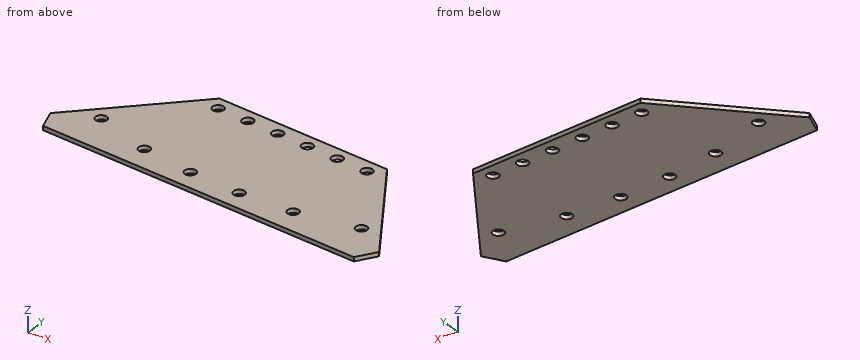
Autodesk Inventor part; units mm, degrees
ref_plane "YZ Plane" through (0, 0, 0) normal (1, 0, 0) x (0, 1, 0)
ref_plane "XZ Plane" through (0, 0, 0) normal (0, 1, 0) x (-1, 0, 0)
ref_plane "XY Plane" through (0, 0, 0) normal (0, 0, 1) x (1, 0, 0)
sketch "Sketch1" plane through (0, 0, 0) normal (0, 0, 1) x (1, 0, 0)
  circle A0 centre (31.6038, 86.1786) radius 2.1844
  circle A1 centre (18.9769, 87.5393) radius 2.1844
  circle A2 centre (6.35, 88.9) radius 2.1844
  circle A3 centre (-6.2769, 90.2607) radius 2.1844
  circle A4 centre (-18.9038, 91.6214) radius 2.1844
  circle A5 centre (-31.5307, 92.9821) radius 2.1844
  line L0 (36.1246, 90.903) -> (-34.9412, 98.5613)
  line L1 (-73.7518, 59.4167) -> (-34.9412, 98.5613)
  line L2 (36.1246, 90.903) -> (65.7044, 44.3885)
  line L3 (61.0548, 36.9038) -> (-70.8037, 51.1132)
  circle A6 centre (52.0487, 54.0287) radius 2.1844
  circle A7 centre (27.7551, 50.4643) radius 2.1844
  circle A8 centre (6.35, 50.8) radius 2.1844
  circle A9 centre (-14.3942, 53.0355) radius 2.1844
  circle A10 centre (-35.3794, 57.2679) radius 2.1844
  circle A11 centre (-58.3558, 65.9262) radius 2.1844
  line L4 (61.0548, 36.9038) -> (65.7044, 44.3885)
  line L5 (-70.8037, 51.1132) -> (-73.7518, 59.4167)
  point P0 (0, 0)
  point P1 (-80.9052, 52.2018)
  point P2 (71.1563, 35.8152)
  dimension "d2" = 10.16
  dimension "d3" = 10.16
  dimension "d4" = 10.16
  dimension "d5" = 10.16
extrude "Extrusion1" add sketch "Sketch1" along normal blind 1.5875
properties part number "Endgame main polycarb"
Work out the finished part from the listing and answer in its coordinate system (mm). Give positions to 0.01 mm unless a question says otherwise; leave off trailing zeros. Write each loop counter-clockwise with the first axis right and the second up, starting at its lowest first coordinate (ties: lowest second). Pieces come first, ordered by that corner, then holes.
(1) The part is cut by section A-A on x = -58.5. Write down the section's boundary in (y, z).
Final values:
outline: (49.79, 0) - (63.75, 0) - (63.75, 1.59) - (49.79, 1.59) - close; (68.11, 0) - (74.8, 0) - (74.8, 1.59) - (68.11, 1.59) - close
(2) The part is cut by section C-C on x = 6.35. Write down the section's boundary in (y, z).
Final values:
outline: (42.8, 0) - (48.62, 0) - (48.62, 1.59) - (42.8, 1.59) - close; (52.98, 0) - (86.72, 0) - (86.72, 1.59) - (52.98, 1.59) - close; (91.08, 0) - (94.11, 0) - (94.11, 1.59) - (91.08, 1.59) - close
(3) A flat-ended cylindrical pin translates along its axis: pin 1 Ø4 at (x, y) = (52.05, 54.03) entering from +Z. Find the tip coordinate at first contact, or state that the pin passes through.
Final values:
pin 1: passes through
(4) Straight lines are drawn through the part: line 1 (X direction, y = 88.5, z = 0.3); line 2 (X direction, y = 54.5, z = 0.3); line 3 (X direction, y = 64.5, z = 1.5). For each, find the intervals that lie inside material, in ascending order.
Final values:
line 1: x = -44.92 to -7.57, -4.98 to 4.2, 8.5 to 17.02, 20.94 to 37.65
line 2: x = -72.01 to -16.01, -12.77 to 49.92, 54.18 to 59.27
line 3: x = -68.71 to -60.01, -56.7 to 52.91
(5) The part is cut by section D-D on y = 74. Write down the section's boundary in (x, z).
Final values:
outline: (-59.29, 0) - (46.87, 0) - (46.87, 1.59) - (-59.29, 1.59) - close
(6) The part is cut by section B-B on z = 0.5. Count the separate pieces of the cut face and the enclosed holes in it, plus the area to 3 significant figures.
Final values:
separate pieces: 1
enclosed holes: 12
area: 5,460 mm2
